Here's how the part is built. I have some questions about the finished solid (model axes, mm). Coordinates: 2 decimals unless noted, no trailing zeros. Write each loop counter-clockwise with the first axis right and the second up, starting at its lowest first coordinate (ties: lowest second). Pieces come first, ordered by that corner, then holes.
Item 1: If we mould it in two halves opening along Y, with no side actions, what happens to faces 1 (the face through (4, 11.5, 11)), 2 (the face through (0, 40, 11)), 3 (the face through (4.717, 13.024, 10.986))? For each: pulls with the +Y half, pulls with the -Y half, needs draft (parallel to the pull), parting line crosses it, or undercut.
Item 2: Please list where these lines run through material, in increasing order: line 1 (Y direction, x = 4.5, z = 11.55); line 2 (X direction, y = 66, z = 11); line 3 (X direction, y = 66.5, z = 11.1).
Item 3: I want a section at A-A (y = 66). Please give me the cut outline in (x, z), and give its area (3 significant figures).
Item 4: I want a section at B-B (x = 4.5). Please give me the cut outline in (y, z).
Autodesk Fusion 360 part; units mm, degrees
sketch "Sketch1" plane through (0, 0, 0) normal (0, 0, 1) x (1, 0, 0)
  line L0 (0, 0) -> (50, 0)
  line L1 (50, 0) -> (50, 80)
  line L2 (50, 80) -> (0, 80)
  line L3 (0, 80) -> (0, 0)
  line L4 (9, 9) -> (41, 9)
  line L5 (41, 9) -> (41, 71)
  line L6 (41, 71) -> (9, 71)
  line L7 (9, 71) -> (9, 9)
  line L8 (2, 62.5) -> (7, 62.5)
  line L9 (7, 62.5) -> (7, 17.5)
  line L10 (7, 17.5) -> (2, 17.5)
  line L11 (2, 17.5) -> (2, 62.5)
  line L12 (0, 40) -> (2, 40)
  line L13 (25, 71) -> (25, 60)
  line L14 (48, 62.5) -> (43, 62.5)
  line L15 (48, 17.5) -> (48, 62.5)
  line L16 (43, 62.5) -> (43, 17.5)
  line L17 (43, 17.5) -> (48, 17.5)
  dimension "d1" = 50
  dimension "d2" = 80
  dimension "d3" = -9
  dimension "d4" = 45
  dimension "d5" = 90
  dimension "d6" = 2
  dimension "d7" = 5
extrude "Extrude1" add sketch "Sketch1" along normal blind 10
sketch "Sketch2" plane through (0, 0, 0) normal (0, 0, -1) x (1, 0, 0)
  line L0 (2, -17.5) -> (7, -17.5)
  line L1 (7, -17.5) -> (7, -62.5)
  line L2 (7, -62.5) -> (2, -62.5)
  line L3 (2, -62.5) -> (2, -17.5)
  line L4 (43, -17.5) -> (48, -17.5)
  line L5 (48, -17.5) -> (48, -62.5)
  line L6 (48, -62.5) -> (43, -62.5)
  line L7 (43, -62.5) -> (43, -17.5)
  line L8 (9, -71) -> (9, -9)
  line L9 (9, -9) -> (41, -9)
  line L10 (41, -9) -> (41, -71)
  line L11 (41, -71) -> (9, -71)
  line L12 (0, 0) -> (0, -80)
  line L13 (0, -80) -> (50, -80)
  line L14 (50, -80) -> (50, 0)
  line L15 (50, 0) -> (0, 0)
  line L16 (0, 0) -> (50, 0)
  line L17 (50, 0) -> (50, -80)
  line L18 (50, -80) -> (0, -80)
  line L19 (0, -80) -> (0, 0)
extrude "Extrude2" add sketch "Sketch2" along normal blind 2 contours L0 L1 L2 L3 | L4 L5 L6 L7 | L12 L13 L14 L15 L16 L17 L18 L19
sketch "Sketch3" plane through (0, 0, 10) normal (0, 0, 1) x (-1, 0, 0)
  line L0 (-7, -17.5) -> (-2, -17.5)
  line L1 (-2, -17.5) -> (-2, -62.5)
  line L2 (-2, -62.5) -> (-7, -62.5)
  line L3 (-7, -62.5) -> (-7, -17.5)
  line L4 (-9, -9) -> (-9, -71)
  line L5 (-9, -71) -> (-41, -71)
  line L6 (-41, -71) -> (-41, -9)
  line L7 (-41, -9) -> (-9, -9)
  line L8 (-48, -17.5) -> (-43, -17.5)
  line L9 (-43, -17.5) -> (-43, -62.5)
  line L10 (-43, -62.5) -> (-48, -62.5)
  line L11 (-48, -62.5) -> (-48, -17.5)
  line L12 (0, -80) -> (0, 0)
  line L13 (0, 0) -> (-50, 0)
  line L14 (-50, 0) -> (-50, -80)
  line L15 (-50, -80) -> (0, -80)
  line L16 (0, -80) -> (-50, -80)
  line L17 (-50, -80) -> (-50, 0)
  line L18 (-50, 0) -> (0, 0)
  line L19 (0, 0) -> (0, -80)
  line L20 (0, -10.5) -> (-50, -10.5)
  line L21 (-50, -10.5) -> (-50, -69.5)
  line L22 (-50, -69.5) -> (0, -69.5)
  line L23 (0, -69.5) -> (0, -10.5)
  line L24 (-4.5, -17.5) -> (-4.5, -10.5)
  line L25 (-4.5, -62.5) -> (-4.5, -69.5)
  line L26 (-45.5, -62.5) -> (-45.5, -69.5)
  line L27 (-45.5, -17.5) -> (-45.5, -10.5)
  circle A0 centre (-4.5, -14) radius 1
  circle A1 centre (-45.5, -14) radius 1
  circle A2 centre (-45.5, -66) radius 1
  circle A3 centre (-4.5, -66) radius 1
  dimension "d12" = 7
  dimension "d13" = 7
  dimension "d14" = 2
  dimension "d15" = 2
  dimension "d16" = 2
  dimension "d17" = 2
extrude "Extrude3" cut sketch "Sketch3" against normal blind 10 contours L24 A0 | L24 A0 | L25 A3 | L25 A3 | L27 A1 | L27 A1 | L26 A2 | L26 A2
extrude "Extrude4" add sketch "Sketch3" along normal blind 2 contours L4 L6 L7 L12 L13 L14 L17 L18 L19 L20 | L4 L5 L6 L12 L14 L15 L16 L17 L19 L22
sketch "Sketch4" plane through (0, 0, 0) normal (0, -1, 0) x (1, 0, 0)
  line L0 (50, -2) -> (50, 12)
  line L1 (50, 12) -> (0, 12)
  line L2 (0, 12) -> (0, -2)
  line L3 (0, -2) -> (50, -2)
  line L4 (25, 12) -> (25, -2)
  circle A0 centre (25, 5) radius 5
  dimension "d22" = 10
extrude "Extrude5" cut sketch "Sketch4" against normal blind 100 contours L4 A0 | L4 A0
sketch "Sketch5" plane through (0, 0, -2) normal (0, 0, -1) x (1, 0, 0)
  line L0 (41, -9) -> (41, -71)
  line L1 (41, -71) -> (9, -71)
  line L2 (9, -71) -> (9, -9)
  line L3 (9, -9) -> (41, -9)
  line L4 (0, -80) -> (50, -80)
  line L5 (50, -80) -> (50, 0)
  line L6 (50, 0) -> (0, 0)
  line L7 (0, 0) -> (0, -80)
  line L8 (10, -80) -> (40, -80)
  line L9 (50, -70) -> (50, -10)
  line L10 (40, 0) -> (10, 0)
  line L11 (0, -10) -> (0, -70)
  line L12 (39.5, -9) -> (10.5, -9)
  line L13 (9, -10.5) -> (9, -69.5)
  line L14 (10.5, -71) -> (39.5, -71)
  line L15 (41, -69.5) -> (41, -10.5)
  arc A0 (10.5, -9) -> (9, -10.5) centre (10.5, -10.5) ccw
  arc A1 (41, -10.5) -> (39.5, -9) centre (39.5, -10.5) ccw
  arc A2 (9, -69.5) -> (10.5, -71) centre (10.5, -69.5) ccw
  arc A3 (39.5, -71) -> (41, -69.5) centre (39.5, -69.5) ccw
  arc A4 (10, 0) -> (0, -10) centre (10, -10) ccw
  arc A5 (50, -10) -> (40, 0) centre (40, -10) ccw
  arc A6 (0, -70) -> (10, -80) centre (10, -70) ccw
  arc A7 (40, -80) -> (50, -70) centre (40, -70) ccw
  point P0 (20, -71)
  point P1 (9, -10.5)
  point P2 (41, -10.5)
  point P3 (41, -69.5)
  point P4 (9, -69.5)
  dimension "d29" = 10
  dimension "d30" = 10
  dimension "d31" = 10
  dimension "d32" = 10
extrude "Extrude6" cut sketch "Sketch5" against normal blind 100 contours L4 L7 A6 | L4 L5 A7 | L6 L7 A4 | L5 L6 A5
extrude "Extrude7" add sketch "Sketch5" against normal up to surface (14 mm away) contours L0 L3 A1 | L0 L1 A3 | L2 L3 A0 | L1 L2 A2
sketch "Sketch6" plane through (0, 0, 10) normal (0, 0, 1) x (-1, 0, 0)
  line L0 (-9, -69.5) -> (0, -69.5)
  line L1 (0, -69.5) -> (0, -10.5)
  line L2 (0, -10.5) -> (-9, -10.5)
  line L3 (-9, -10.5) -> (-9, -69.5)
  line L4 (-7, -17.5) -> (-2, -17.5)
  line L5 (-2, -17.5) -> (-2, -62.5)
  line L6 (-2, -62.5) -> (-7, -62.5)
  line L7 (-7, -62.5) -> (-7, -17.5)
  circle A0 centre (-4.5, -66) radius 1
  circle A1 centre (-4.5, -14) radius 1
  line L8 (0, -69.5) -> (-9, -69.5)
  line L9 (-9, -69.5) -> (-9, -10.5)
  line L10 (-9, -10.5) -> (0, -10.5)
  line L11 (0, -10.5) -> (0, -69.5)
  line L12 (12.8472, -89.0472) -> (-65.8375, -89.0472)
  line L13 (-65.8375, -89.0472) -> (-65.8375, 10.3586)
  line L14 (-65.8375, 10.3586) -> (12.8472, 10.3586)
  line L15 (12.8472, 10.3586) -> (12.8472, -89.0472)
extrude "Extrude8" cut sketch "Sketch6" against normal blind 100 from surface at 2 contours L12 L13 L14 L15
sketch "Sketch7" plane through (0, 0, 10) normal (0, 0, 1) x (-1, 0, 0)
  line L0 (-9, -69.5) -> (0, -69.5)
  line L1 (0, -69.5) -> (0, -10.5)
  line L2 (0, -10.5) -> (-9, -10.5)
  line L3 (-9, -10.5) -> (-9, -69.5)
  line L4 (-7, -17.5) -> (-2, -17.5)
  line L5 (-2, -17.5) -> (-2, -62.5)
  line L6 (-2, -62.5) -> (-7, -62.5)
  line L7 (-7, -62.5) -> (-7, -17.5)
  circle A0 centre (-4.5, -66) radius 1
  circle A1 centre (-4.5, -14) radius 1
  line L8 (0, -69.5) -> (-9, -69.5)
  line L9 (-9, -69.5) -> (-9, -10.5)
  line L10 (-9, -10.5) -> (0, -10.5)
  line L11 (0, -10.5) -> (0, -69.5)
extrude "Extrude9" add sketch "Sketch7" along normal blind 2 contours L0 L1 L2 L3 L8 L9 L10 L11 | L4 L5 L6 L7
sketch "Sketch8" plane through (0, 0, 0) normal (-1, 0, 0) x (0, -1, 0)
  line L0 (-10.5, -2) -> (-10.5, 12)
  line L1 (-10.5, 12) -> (-69.5, 12)
  line L2 (-69.5, 12) -> (-69.5, -2)
  line L3 (-69.5, -2) -> (-10.5, -2)
  line L4 (-69.5, -2) -> (-10.5, -2)
  line L5 (-10.5, -2) -> (-10.5, 10)
  line L6 (-10.5, 10) -> (-69.5, 10)
  line L7 (-69.5, 10) -> (-69.5, -2)
  dimension "d42" = 2
extrude "Extrude10" cut sketch "Sketch8" against normal blind 9 contours L0 L2 L3 L4 L5 L6 L7
extrude "Extrude11" cut 1 faces at (3, 10.5, 11.3333) along direction (0, 1, 0) blind 1
extrude "Extrude12" cut 1 faces at (6, 69.5, 11.3333) along direction (0, -1, 0) blind 1
Answer:
1. face 1: pulls with the -Y half
1. face 2: needs draft
1. face 3: undercut
2. line 1: y = 11.5 to 13, 15 to 65, 67 to 68.5
2. line 2: x = 0 to 3.5, 5.5 to 9
2. line 3: x = 0 to 3.63, 5.37 to 9
3. outline: (0, 10) - (3.5, 10) - (3.5, 12) - (0, 12) - close; (5.5, 10) - (9, 10) - (9, 12) - (5.5, 12) - close
3. area: 14.0 mm2
4. outline: (11.5, 10) - (13, 10) - (13, 12) - (11.5, 12) - close; (15, 10) - (65, 10) - (65, 12) - (15, 12) - close; (67, 10) - (68.5, 10) - (68.5, 12) - (67, 12) - close
